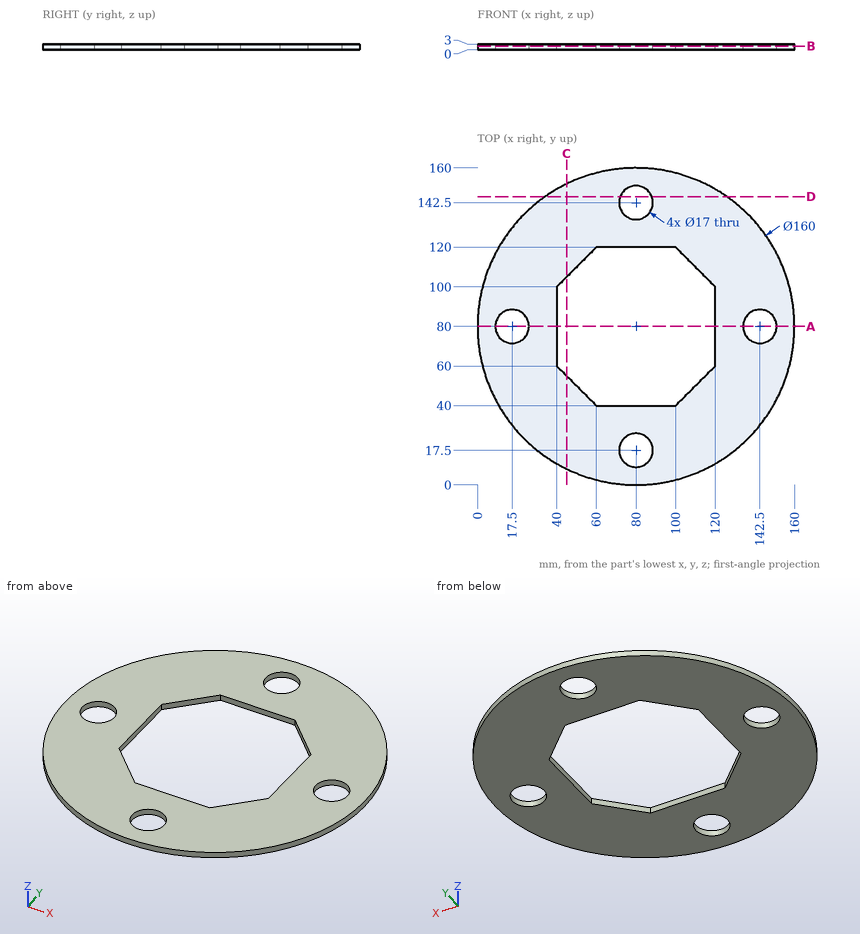
Can you work these out from the drawing? Everything is in mm from the part's minimum corner. Give positions to 0.01 mm unless a question says otherwise; leave off trailing zeros. Order: outer loops, then holes, each group sorted by start corner. A loop starts at its lowest first (then second) coordinate and runs counter-clockwise, first axis right, second up.
Item 1: If we section it at A-A, the plane y = 80: Write out the boundary of the cut face in (x, z).
Item 2: If we section it at D-D, the plane y = 145.5: Write out the boundary of the cut face in (x, z).
Item 3: If we section it at C-C, the plane x = 45: Write out the boundary of the cut face in (y, z), plus the area to 3 significant figures.
Item 4: I need wall thicknesses on line 1 (Y direction, x = 80, z = 1.5); line 2 (Y direction, x = 85.5, z = 0.25); line 3 (X direction, y = 144.5, z = 2). Which ranges of each line are inside material? Lowest first, please.
Item 5: If we section it at B-B, the plane z = 1.9: Write out the boundary of the cut face in (x, y), plus the area to 3 significant figures.
Item 6: I'm going to push flat-ended pins straight in: pin 1 (1.5 mm diameter, centred on x = 118, z = 2.5, fed in from +Y); pin 2 (0.9 mm diameter, centred on x = 83.5, z = 1.5, fed in from +Y). Where does each tip first touch, or does it pass through?
Values:
1. outline: (0, 0) - (9, 0) - (9, 3) - (0, 3) - close; (26, 0) - (40, 0) - (40, 3) - (26, 3) - close; (120, 0) - (134, 0) - (134, 3) - (120, 3) - close; (151, 0) - (160, 0) - (160, 3) - (151, 3) - close
2. outline: (34.07, 0) - (72.05, 0) - (72.05, 3) - (34.07, 3) - close; (87.95, 0) - (125.93, 0) - (125.93, 3) - (87.95, 3) - close
3. outline: (8.06, 0) - (55, 0) - (55, 3) - (8.06, 3) - close; (105, 0) - (151.94, 0) - (151.94, 3) - (105, 3) - close
3. area: 282 mm2
4. line 1: y = 0 to 9, 26 to 40, 120 to 134, 151 to 160
4. line 2: y = 0.19 to 11.02, 23.98 to 40, 120 to 136.02, 148.98 to 159.81
4. line 3: x = 32.67 to 71.74, 88.26 to 127.33
5. outline: circle Ø160 at (80, 80); hole circle Ø17 at (17.5, 80); hole (40, 60) - (60, 40) - (100, 40) - (120, 60) - (120, 100) - (100, 120) - (60, 120) - (40, 100) - close; hole circle Ø17 at (80, 17.5); hole circle Ø17 at (80, 142.5); hole circle Ø17 at (142.5, 80)
5. area: 13,600 mm2
6. pin 1: stops at y = 150.8
6. pin 2: stops at y = 159.94
